Autodesk Inventor part; units mm, degrees
ref_plane "YZ Plane" through (0, 0, 0) normal (1, 0, 0) x (0, 1, 0)
ref_plane "XZ Plane" through (0, 0, 0) normal (0, 1, 0) x (-1, 0, 0)
ref_plane "XY Plane" through (0, 0, 0) normal (0, 0, 1) x (1, 0, 0)
sketch "Boceto1" plane through (0, 0, 0) normal (0, 1, 0) x (-1, 0, 0)
  line L0 (5, 40) -> (-5, 40)
  line L1 (-5, 40) -> (-5, -40)
  line L2 (-5, -40) -> (5, -40)
  line L3 (5, -40) -> (5, 40)
  line L4 (5, 40) -> (-5, -40) construction
  line L5 (-5, 40) -> (5, -40) construction
  circle A0 centre (0, 35) radius 3
  circle A1 centre (0, -35) radius 3
  point P0 (0, 0)
  dimension "d0" = 10
  dimension "d1" = 80
  dimension "d2" = 6
  dimension "d3" = 6
  dimension "d4" = 5
  dimension "d5" = 5
extrude "Extrusión1" add sketch "Boceto1" along normal mid plane 5
fillet "Empalme1" radius 5 4 edges at (-5, 0, 40) (5, 0, 40) (5, 0, -40) (-5, 0, -40)
properties material "Titanio"
Geometry: final body of the model. Coordinates: model frame, mm. Round coordinates to 2 decimals unless told otherwise and drop trailing zeros. Loops run counter-clockwise (first coordinate to the right, second up) from the corner with the lowest first, then second, coordinate; pieces in that order, holes last. Notation, with made-up numbers: (65.5, 58) -> (110.5, 58) arc R25 ccw to (110.5, 88) -> close; hole circle Ø4 at (-12, 86). An arc over 180 degrees is marked (long way). Write each question's results on one line, items separated by ' | '.
Item 1: Cut plane A-A on y = 0.15. State how many separate pieces and enclosed holes the cut face has, and give its area (3 significant figures).
Answers below:
separate pieces: 1 | enclosed holes: 2 | area: 722 mm²
Item 2: Pin query (flat end, axial travel): pin 1 Ø1.5 at (x, y) = (-4, -2) entering from +Z. Return the tip coordinate at first contact, or that it passes through.
Answers below:
pin 1: stops at z = 38.8
Item 3: Cut plane C-C on x = -3.75. Return the cut outline in (y, z).
Answers below:
outline: (-2.5, -38.31) -> (2.5, -38.31) -> (2.5, 38.31) -> (-2.5, 38.31) -> close
Item 4: Cut plane B-B on x = 2. Return the cut outline in (y, z).
Answers below:
outline: (-2.5, -39.58) -> (2.5, -39.58) -> (2.5, -37.24) -> (-2.5, -37.24) -> close; (-2.5, -32.76) -> (2.5, -32.76) -> (2.5, 32.76) -> (-2.5, 32.76) -> close; (-2.5, 37.24) -> (2.5, 37.24) -> (2.5, 39.58) -> (-2.5, 39.58) -> close
Item 5: Line query: probe 1 along Z at (x, y) = (0, -1); probe 2 along Z at (x, y) = (-1, -0.95); probe 3 along Z at (x, y) = (4, -0.35). Output: solid intervals per line, ascending. Write a range as [from, to].
Answers below:
probe 1: z = [-40, -38], [-32, 32], [38, 40] | probe 2: z = [-39.9, -37.83], [-32.17, 32.17], [37.83, 39.9] | probe 3: z = [-38, 38]
Item 6: Pull-direction query (X, two-part tool) for faces 1 (the face through (0, 0, -38)), 2 (the face through (0, 0, 32)), 3 (the face through (3, 0, -39)), 4 (the face through (-4, 0, 38)); classes: pulls with the +X half, pulls with the -X half, needs draft (parallel to the pull), parting line crosses it, or undercut.
Answers below:
face 1: undercut | face 2: undercut | face 3: pulls with the +X half | face 4: pulls with the -X half
